For this review, take the finished solid that the model builds, in its own axes (mm). A direction names the side the tool comes from. Give positions to 0.01 mm unless a question says otherwise; leave off trailing zeros. Order: outer loops, then holes, each group sorted by start corner. A loop starts at its lowest first (then second) coordinate and runs counter-clockwise, first axis right, second up. Notation, with made-up numbers: M 58.25,56.5 L 89.25,56.5 A18 cw 89.25,87.5 Z; hole C -26,21.5 d1. An arc over 180 degrees is marked long. Answer as CSV lines item,"result". Start each with the question number.
1. For line 1 along Z through (x, y) = (71.5, 60); line 2 along Y through (x, z) = (47, 1); line 3 along Z through (x, y) = (48.5, 46.5), list the stretches that pass through material, from the lowest coordinate up.
2. We need section A-A, the plane y = 14.5. Give the boundary of the cut face in (x, z), and give its area (3 significant figures).
3. Mouldability with a two-part tool opening along Y and no side actions: class faces 1 (the flat face through (74, 65, 3)), 2 (the flat face through (74, 37, 0)), 3 (the flat face through (95, 46, -37.65)) as pulls with the +Y half, pulls with the -Y half, needs draft (parallel to the pull), parting line crosses it, or undercut.
4. We need section C-C, the plane x = 31.5. Give the boundary of the cut face in (y, z).
5. We need section B-B, the plane x = 138.5. Give the boundary of the cut face in (y, z).
6. We need section D-D, the plane y = 44. State how many separate pieces and enclosed holes the cut face has, and give its area (3 significant figures).
7. Machinability: for faces 4 (the flat face through (140, 46, -37.65)), 5 (the cylindrical face through (92.48, 4.78, 3.55)), 6 (the cylindrical face through (136.302, 44.097, -38.537)), which of the approach directions +Z, -Z, +X, -X, +Y, -Y give a long, thin tool a straight path to every point of the face, cutting with its end or side? Answer none if there is none.
8. Clearance check with flat-ended pins moving along their axes: P1, Ø10, axis at x = 73, z = -11.5, coming from the +Y side; P2, Ø2.5, axis at x = 59.5, y = 4.5, coming from the +Z side. State where each tip first meets the part, or that it passes through.
from build123d import *

# Parameters (mm, degrees)
SKETCH1_W           = 150
SKETCH1_H           = 65
BOSS_EXTRUDE1_DEPTH = 7
CUT_EXTRUDE1_REACH  = 165.628
SKETCH2_R           = 2.2
SKETCH3_W           = 150
SKETCH3_H           = 8
BOSS_EXTRUDE2_DEPTH = 16.2
SKETCH4_R           = 6.6
CUT_EXTRUDE2_DEPTH  = 5.25
CHAMFER1_SIZE       = 0.5
SKETCH5_R           = 2.6
CUT_EXTRUDE3_DEPTH  = 7
SKETCH7_R           = 1.5
CUT_EXTRUDE4_DEPTH  = 169.158734534


with BuildPart() as part:
    # Sketch1 → Boss-Extrude1 (new body)
    with BuildSketch(Plane.XY):
        with Locations((75, 32.5)):
            Rectangle(SKETCH1_W, SKETCH1_H)
    boss_extrude1 = extrude(amount=BOSS_EXTRUDE1_DEPTH)

    # Sketch2 → Cut-Extrude1 (cut, up to next)
    with BuildSketch(Plane.XY.offset(7), mode=Mode.PRIVATE) as cut_extrude1_sk1:
        with Locations((10, 44)):
            Circle(SKETCH2_R)
    cut_extrude1_tool1 = extrude(cut_extrude1_sk1.sketch, amount=-CUT_EXTRUDE1_REACH, mode=Mode.PRIVATE) & part.part
    # Sketch2 → Cut-Extrude1 (cut, up to next)
    with BuildSketch(Plane.XY.offset(7), mode=Mode.PRIVATE) as cut_extrude1_sk2:
        with Locations((47.5, 44)):
            Circle(SKETCH2_R)
    cut_extrude1_tool2 = extrude(cut_extrude1_sk2.sketch, amount=-CUT_EXTRUDE1_REACH, mode=Mode.PRIVATE) & part.part
    # Sketch2 → Cut-Extrude1 (cut, up to next)
    with BuildSketch(Plane.XY.offset(7), mode=Mode.PRIVATE) as cut_extrude1_sk3:
        with Locations((93, 44)):
            Circle(SKETCH2_R)
    cut_extrude1_tool3 = extrude(cut_extrude1_sk3.sketch, amount=-CUT_EXTRUDE1_REACH, mode=Mode.PRIVATE) & part.part
    # Sketch2 → Cut-Extrude1 (cut, up to next)
    with BuildSketch(Plane.XY.offset(7), mode=Mode.PRIVATE) as cut_extrude1_sk4:
        with Locations((138.5, 44)):
            Circle(SKETCH2_R)
    cut_extrude1_tool4 = extrude(cut_extrude1_sk4.sketch, amount=-CUT_EXTRUDE1_REACH, mode=Mode.PRIVATE) & part.part
    cut_extrude1_1 = cut_extrude1_tool1.solids().sort_by_distance((10, 44, 7))[0]
    add(cut_extrude1_1, mode=Mode.SUBTRACT)
    cut_extrude1_2 = cut_extrude1_tool2.solids().sort_by_distance((47.5, 44, 7))[0]
    add(cut_extrude1_2, mode=Mode.SUBTRACT)
    cut_extrude1_3 = cut_extrude1_tool3.solids().sort_by_distance((93, 44, 7))[0]
    add(cut_extrude1_3, mode=Mode.SUBTRACT)
    cut_extrude1_4 = cut_extrude1_tool4.solids().sort_by_distance((138.5, 44, 7))[0]
    add(cut_extrude1_4, mode=Mode.SUBTRACT)
    cut_extrude1 = cut_extrude1_1 + cut_extrude1_2 + cut_extrude1_3 + cut_extrude1_4  # Cut-Extrude1 as one shape, for the pattern or mirror that repeats it

    # Sketch3 → Boss-Extrude2 (add)
    with BuildSketch(Plane(origin=(0, 0, 0), x_dir=(-1, 0, 0), z_dir=(0, 0, -1))):
        with Locations((-75, 4)):
            Rectangle(SKETCH3_W, SKETCH3_H)
    boss_extrude2 = extrude(amount=BOSS_EXTRUDE2_DEPTH)

    # Sketch4 → Cut-Extrude2 (cut)
    with BuildSketch(Plane(origin=(0, 0, 0), x_dir=(-1, 0, 0), z_dir=(0, 0, -1))):
        with Locations((-138.5, 44)):
            Circle(SKETCH4_R)
        with Locations((-93, 44)):
            Circle(SKETCH4_R)
        with Locations((-47.5, 44)):
            Circle(SKETCH4_R)
        with Locations((-10, 44)):
            Circle(SKETCH4_R)
    cut_extrude2 = extrude(amount=-CUT_EXTRUDE2_DEPTH, mode=Mode.SUBTRACT)

    # Mirror2: Boss-Extrude2 across plane
    add(boss_extrude2.mirror(Plane.XY.offset(-16.2)))

    # Mirror3: Boss-Extrude1, Cut-Extrude1, Cut-Extrude2 across plane
    add(boss_extrude1.mirror(Plane(origin=(0, 0, -16.2), x_dir=(1, 0, 0), z_dir=(0, 0, -1))))
    add(cut_extrude1.mirror(Plane(origin=(0, 0, -16.2), x_dir=(1, 0, 0), z_dir=(0, 0, -1))), mode=Mode.SUBTRACT)
    add(cut_extrude2.mirror(Plane(origin=(0, 0, -16.2), x_dir=(1, 0, 0), z_dir=(0, 0, -1))), mode=Mode.SUBTRACT)

    # Chamfer1
    chamfer1_edges = [part.edges().sort_by_distance(p)[0] for p in [
        (145.1, 44, -32.4),
        (99.6, 44, -32.4),
        (54.1, 44, -32.4),
        (16.6, 44, -32.4),
        (145.1, 44, 0),
        (99.6, 44, 0),
        (54.1, 44, 0),
        (16.6, 44, 0),
    ]]
    chamfer(chamfer1_edges, length=CHAMFER1_SIZE)

    # Sketch5 → Cut-Extrude3 (cut)
    with BuildSketch(Plane.XY.offset(7)):
        with Locations((60.000022648, 4.052132501)):
            Circle(SKETCH5_R)
        with Locations((89.999977352, 4)):
            Circle(SKETCH5_R)
    extrude(amount=-CUT_EXTRUDE3_DEPTH, mode=Mode.SUBTRACT)

    # Sketch7 → Cut-Extrude4 (cut, through all)
    with BuildSketch(Plane.XY):
        with Locations((60.000022648, 4.052132501)):
            Circle(SKETCH7_R)
        with Locations((89.999977352, 4)):
            Circle(SKETCH7_R)
    extrude(amount=-CUT_EXTRUDE4_DEPTH, mode=Mode.SUBTRACT)


solid = part.part
Result set:
1,line 1,"-39.4 to -32.4, 0 to 7"
1,line 2,"0 to 37.42, 50.58 to 65"
1,line 3,"-39.4 to -37.65, 5.25 to 7"
2,outline,"M 0,-39.4 L 150,-39.4 L 150,-32.4 L 0,-32.4 Z; M 0,0 L 150,0 L 150,7 L 0,7 Z"
2,area,"2,100 mm2"
3,face 1,"pulls with the +Y half"
3,face 2,"needs draft"
3,face 3,"undercut"
4,outline,"M 0,-39.4 L 65,-39.4 L 65,-32.4 L 8,-32.4 L 8,0 L 65,0 L 65,7 L 0,7 Z"
5,outline,"M 0,-39.4 L 41.8,-39.4 L 41.8,-37.65 L 37.4,-37.65 L 37.4,-32.9 L 36.9,-32.4 L 8,-32.4 L 8,0 L 36.9,0 L 37.4,0.5 L 37.4,5.25 L 41.8,5.25 L 41.8,7 L 0,7 Z; M 46.2,-39.4 L 65,-39.4 L 65,-32.4 L 51.1,-32.4 L 50.6,-32.9 L 50.6,-37.65 L 46.2,-37.65 Z; M 46.2,5.25 L 50.6,5.25 L 50.6,0.5 L 51.1,0 L 65,0 L 65,7 L 46.2,7 Z"
6,separate pieces,"10"
6,enclosed holes,"0"
6,area,"1,480 mm2"
7,face 4,"none"
7,face 5,"+Z"
7,face 6,"+Z, -Z"
8,P1,"y = 8"
8,P2,"z = 0"
